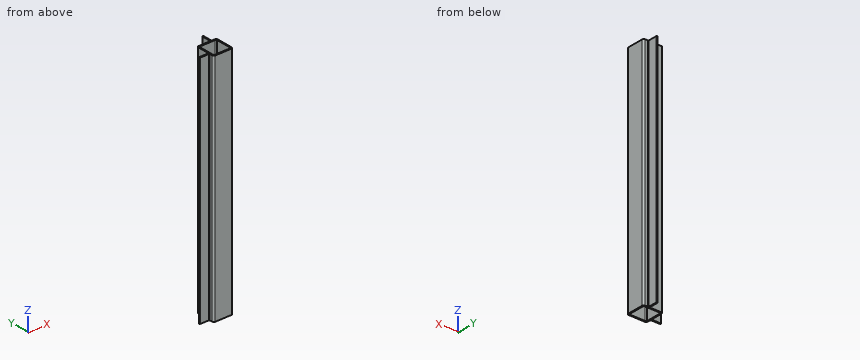
Autodesk Inventor part; units mm, degrees
ref_plane "YZ Plane" through (0, 0, 0) normal (1, 0, 0) x (0, 1, 0)
ref_plane "XZ Plane" through (0, 0, 0) normal (0, 1, 0) x (-1, 0, 0)
ref_plane "XY Plane" through (0, 0, 0) normal (0, 0, 1) x (1, 0, 0)
sketch "Sketch1" plane through (0, 0, 0) normal (0, 0, 1) x (1, 0, 0)
  line L0 (11.176, -9.652) -> (11.176, 9.652)
  arc A0 (9.652, -11.176) -> (11.176, -9.652) centre (9.652, -9.652) ccw
  line L1 (-9.652, -11.176) -> (9.652, -11.176)
  arc A1 (-11.176, -9.652) -> (-9.652, -11.176) centre (-9.652, -9.652) ccw
  line L2 (-11.176, 9.652) -> (-11.176, -9.652)
  arc A2 (-9.652, 11.176) -> (-11.176, 9.652) centre (-9.652, 9.652) ccw
  line L3 (9.652, 11.176) -> (-9.652, 11.176)
  arc A3 (11.176, 9.652) -> (9.652, 11.176) centre (9.652, 9.652) ccw
  arc A4 (6.35, 13.462) -> (7.112, 12.7) centre (7.112, 13.462) ccw
  line L4 (6.35, 13.462) -> (6.35, 24.638)
  arc A5 (6.35, 24.638) -> (4.826, 24.638) centre (5.588, 24.638) ccw
  line L5 (4.826, 24.638) -> (4.826, 13.462)
  arc A6 (4.064, 12.7) -> (4.826, 13.462) centre (4.064, 13.462) ccw
  line L6 (4.064, 12.7) -> (-10.5918, 12.7)
  arc A7 (-10.5918, 12.7) -> (-12.7, 10.5918) centre (-10.5918, 10.5918) ccw
  line L7 (-12.7, 10.5918) -> (-12.7, -4.064)
  arc A8 (-13.462, -4.826) -> (-12.7, -4.064) centre (-13.462, -4.064) ccw
  line L8 (-13.462, -4.826) -> (-24.638, -4.826)
  arc A9 (-24.638, -4.826) -> (-24.638, -6.35) centre (-24.638, -5.588) ccw
  line L9 (-24.638, -6.35) -> (-13.462, -6.35)
  arc A10 (-12.7, -7.112) -> (-13.462, -6.35) centre (-13.462, -7.112) ccw
  line L10 (-12.7, -7.112) -> (-12.7, -10.5918)
  arc A11 (-12.7, -10.5918) -> (-10.5918, -12.7) centre (-10.5918, -10.5918) ccw
  line L11 (-10.5918, -12.7) -> (10.5918, -12.7)
  arc A12 (10.5918, -12.7) -> (12.7, -10.5918) centre (10.5918, -10.5918) ccw
  line L12 (12.7, -10.5918) -> (12.7, 10.5918)
  arc A13 (12.7, 10.5918) -> (10.5918, 12.7) centre (10.5918, 10.5918) ccw
  line L13 (10.5918, 12.7) -> (7.112, 12.7)
  point P0 (0, 0)
extrude "Extrusion1" add sketch "Sketch1" against normal blind 304.8
properties part number "9010"
Source: CAD feature listing. Evaluate the final solid. Frame: model axes, mm. Round coordinates to 2 decimals unless told otherwise and drop trailing zeros. Loops run counter-clockwise (first coordinate to the right, second up) from the corner with the lowest first, then second, coordinate; pieces in that order, holes last. Notation, with made-up numbers: M 2,15.25 L 38,15.25 A28 cw 38,39.25 Z; hole C -23,-17 d1. An arc over 180 degrees is marked long. Return JSON: item names as keys, results as strings. Group by question number.
1. Section query D-D on x = -19. Output: boundary loops of the cut face in (y, z).
2. Material intervals for line 1 along X through (y, z) = (2, -219); line 2 along X through (y, z) = (14, -31), sorted ascending. Write a range as from..to.
3. Section query A-A on x = -2. Output: boundary loops of the cut face in (y, z).
4. Section query C-C on z = -248.5. Output: boundary loops of the cut face in (x, y).
5. Pin query (flat end, axial travel): pin 1 (1.7 mm diameter, centred on y = -9, z = -138, fed in from -X); pin 2 (6 mm diameter, centred on y = 18.5, z = -209, fed in from +X); pin 3 (1 mm diameter, centred on x = -11, z = -233.5, fed in from +Y). Return the tip coordinate at first contact, or that it passes through.
Checks:
{
 "1": {"outline": "M -6.35,-304.8 L -4.83,-304.8 L -4.83,0 L -6.35,0 Z"},
 "2": {"line 1": "x = -12.7..-11.18, 11.18..12.7", "line 2": "x = 4.83..6.35"},
 "3": {"outline": "M -12.7,-304.8 L -11.18,-304.8 L -11.18,0 L -12.7,0 Z; M 11.18,-304.8 L 12.7,-304.8 L 12.7,0 L 11.18,0 Z"},
 "4": {"outline": "M -24.64,-6.35 L -13.46,-6.35 A0.76 cw -12.7,-7.11 L -12.7,-10.59 A2.11 ccw -10.59,-12.7 L 10.59,-12.7 A2.11 ccw 12.7,-10.59 L 12.7,10.59 A2.11 ccw 10.59,12.7 L 7.11,12.7 A0.76 cw 6.35,13.46 L 6.35,24.64 A0.76 ccw 4.83,24.64 L 4.83,13.46 A0.76 cw 4.06,12.7 L -10.59,12.7 A2.11 ccw -12.7,10.59 L -12.7,-4.06 A0.76 cw -13.46,-4.83 L -24.64,-4.83 A0.76 ccw Z; hole M -11.18,-9.65 A1.52 ccw -9.65,-11.18 L 9.65,-11.18 A1.52 ccw 11.18,-9.65 L 11.18,9.65 A1.52 ccw 9.65,11.18 L -9.65,11.18 A1.52 ccw -11.18,9.65 Z"},
 "5": {"pin 1": "stops at x = -12.7", "pin 2": "stops at x = 6.35", "pin 3": "stops at y = 12.7"}
}
